Can you work these out from the drawing? Everything is in mm from the part's minimum corner. A direction names the side the tool comes from. Coordinates: 2 decimals unless noted, no trailing zeros. Loops run counter-clockwise (first coordinate to the right, second up) from the corner with the lowest first, then second, coordinate; pieces in that order, holes last. Notation, with made-up numbers: (3.25, 2) - (41.25, 2) arc R8 cw to (41.25, 7) - close; hole circle Ø3 at (-20, 71). An arc over 180 degrees is marked (long way). Put each result on its own line as item: value. Start each with the question number.
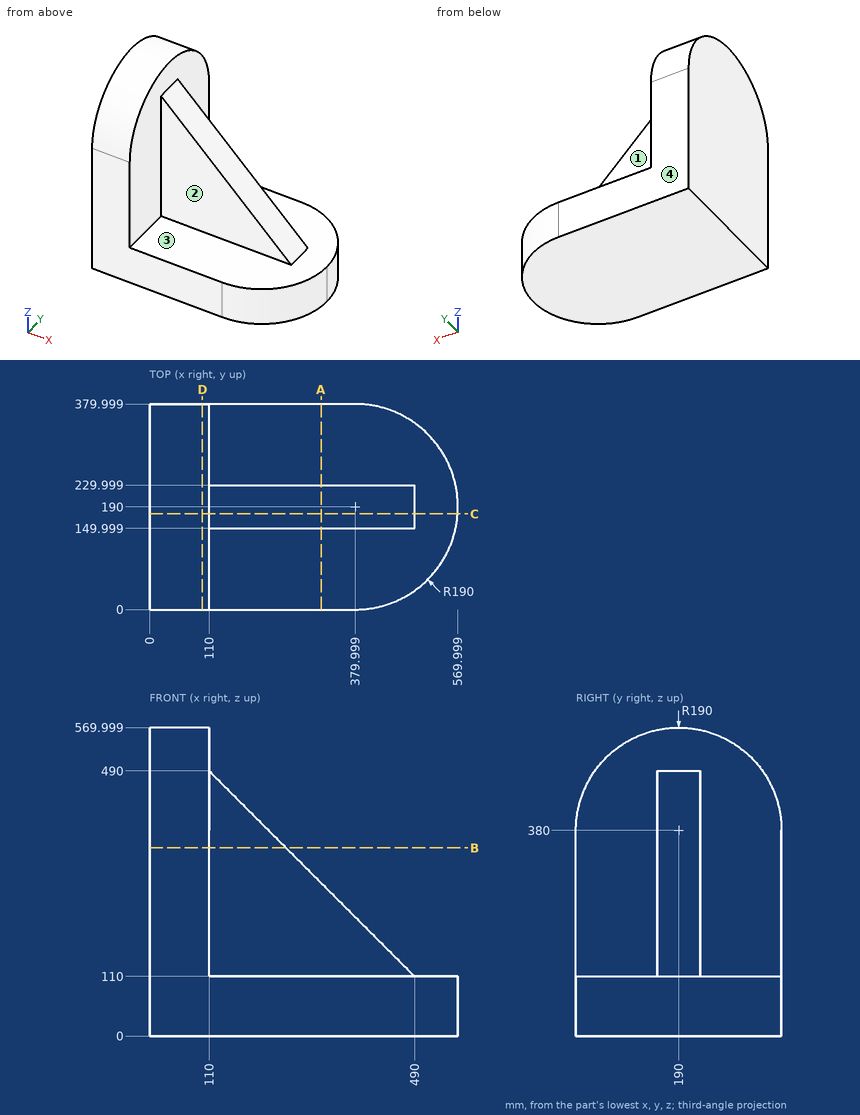
Q1. I want a section at D-D on x = 97.5. List the corners of the cut face in (y, z) for me.
Q2. On a 3-axis mill with a long thin cutter (end or side, diameter ignored), from which of +Z, -Z, +X, -X, +Y, -Y can I reach the whole of each face in a straight line? I mean the marked faces 1, 2, 3 and 4. Say none if no direction works.
Q3. Will these pins go through, and if not, where does the flat tip stop? pin 1 (1 mm diameter, centred on y = 156.5, z = 304, fed in from +X); pin 2 (3 mm diameter, centred on x = 435, y = 187, fed in from +Z); pin 3 (1.5 mm diameter, centred on x = 106, y = 71, fed in from +Z).
Q4. I want a section at A-A on x = 317. List the corners of the cut face in (y, z) for me, and give its area (3 significant figures).
Q5. Please list where these lines run through material, in increasing order: line 1 along X through (y, z) = (356, 461.5); line 2 along Y through (x, z) = (313, 149.5). Write a range as [from, to].
Q6. I want a section at C-C on y = 177. List the corners of the cut face in (x, z) for me.
Q7. I want a section at B-B on z = 347.5. List the corners of the cut face in (x, y) for me.
Calculated:
1. outline: (0, 0) - (380, 0) - (380, 380) arc R190 ccw to (0, 380) - close
2. face 1: +Z, +X, +Y
2. face 2: +Z, +X, -Y
2. face 3: +Z, +X
2. face 4: +Z, -Z, +X, -X, +Y
3. pin 1: x = 296.5
3. pin 2: z = 166.5
3. pin 3: z = 528.72
4. outline: (0, 0) - (380, 0) - (380, 110) - (230, 110) - (230, 283) - (150, 283) - (150, 110) - (0, 110) - close
4. area: 55,600 mm2
5. line 1: [0, 110]
5. line 2: [150, 230]
6. outline: (0, 0) - (569.55, 0) - (569.55, 110) - (490, 110) - (110, 490) - (110, 569.55) - (0, 569.55) - close
7. outline: (0, 0) - (110, 0) - (110, 150) - (252.5, 150) - (252.5, 230) - (110, 230) - (110, 380) - (0, 380) - close
